Design review of the part built by this model. Coordinates are the model's own, in mm. A direction names the side the tool comes from. Give positions to 0.01 mm unless a question says otherwise; leave off trailing zeros. Write each loop counter-clockwise with the first axis right and the second up, starting at its lowest first coordinate (ties: lowest second). Pieces come first, ordered by that corner, then holes. Notation, with made-up numbers: (-7, -38.5) -> (35, -38.5) arc R21 cw to (35, -22.5) -> close; hole circle Ø5 at (-18.75, -12.75). An arc over 180 degrees is marked (long way). Put each result on its own line as item: value. Start each with the question number.
from build123d import *

# Parameters (mm, degrees)
SKETCH1_R           = 13
BOSS_EXTRUDE1_DEPTH = 17.5
SKETCH6_R           = 5
BOSS_EXTRUDE2_DEPTH = 6
SKETCH7_R           = 5.5
BOSS_EXTRUDE3_DEPTH = 0.5
SKETCH2_R           = 1.65
CUT_EXTRUDE1_DEPTH  = 24.5
CUT_EXTRUDE3_START  = -4
SKETCH5_R           = 3.55
CUT_EXTRUDE3_DEPTH  = 11
CIRPATTERN1_COUNT   = 4
SKETCH3_R           = 2.05
CUT_EXTRUDE2_DEPTH  = 24.5
SKETCH8_R           = 2.75
CUT_EXTRUDE4_DEPTH  = 10
CUT_EXTRUDE5_DEPTH  = 10


with BuildPart() as part:
    # Sketch1 → Boss-Extrude1 (new body)
    with BuildSketch(Plane(origin=(0, 0, 0), x_dir=(1, 0, 0), z_dir=(0, 1, 0))):
        Circle(SKETCH1_R)
    extrude(amount=BOSS_EXTRUDE1_DEPTH)

    # Sketch6 → Boss-Extrude2 (add)
    with BuildSketch(Plane(origin=(0, 17.5, 0), x_dir=(1, 0, 0), z_dir=(0, 1, 0))):
        with Locations((1, 0)):
            Circle(SKETCH6_R)
    extrude(amount=BOSS_EXTRUDE2_DEPTH)

    # Sketch7 → Boss-Extrude3 (add)
    with BuildSketch(Plane(origin=(0, 17.5, 0), x_dir=(1, 0, 0), z_dir=(0, 1, 0))):
        with Locations((1, 0)):
            Circle(SKETCH7_R)
    extrude(amount=BOSS_EXTRUDE3_DEPTH)

    # Sketch2 → Cut-Extrude1 (cut, through all)
    with BuildSketch(Plane(origin=(0, 0, 0), x_dir=(1, 0, 0), z_dir=(0, 1, 0))):
        with Locations((0, 9)):
            Circle(SKETCH2_R)
    cut_extrude1 = extrude(amount=CUT_EXTRUDE1_DEPTH, mode=Mode.SUBTRACT)

    # Sketch5 → Cut-Extrude3 (cut)
    with BuildSketch(Plane(origin=(0, 17.5, 0), x_dir=(1, 0, 0), z_dir=(0, 1, 0)).offset(CUT_EXTRUDE3_START)):
        with Locations((0, 9)):
            Circle(SKETCH5_R)
    cut_extrude3 = extrude(amount=CUT_EXTRUDE3_DEPTH, mode=Mode.SUBTRACT)

    # CirPattern1: Cut-Extrude1, Cut-Extrude3 ×4 about axis
    cirpattern1_axis = Axis((0, 0, 0), (0, 1, 0))
    for i in range(1, CIRPATTERN1_COUNT):
        add(cut_extrude1.rotate(cirpattern1_axis, i * 360 / CIRPATTERN1_COUNT), mode=Mode.SUBTRACT)
        add(cut_extrude3.rotate(cirpattern1_axis, i * 360 / CIRPATTERN1_COUNT), mode=Mode.SUBTRACT)

    # Sketch3 → Cut-Extrude2 (cut, through all)
    with BuildSketch(Plane(origin=(0, 0, 0), x_dir=(1, 0, 0), z_dir=(0, 1, 0))):
        Circle(SKETCH3_R)
    extrude(amount=CUT_EXTRUDE2_DEPTH, mode=Mode.SUBTRACT)

    # Sketch8 → Cut-Extrude4 (cut)
    with BuildSketch(Plane.XZ):
        Circle(SKETCH8_R)
    extrude(amount=-CUT_EXTRUDE4_DEPTH, mode=Mode.SUBTRACT)

    # Sketch10 → Cut-Extrude5 (cut)
    with BuildSketch(Plane.XZ):
        Polygon((4.618802154, 0), (2.309401077, 4), (-2.309401077, 4), (-4.618802154, 0), (-2.309401077, -4), (2.309401077, -4), align=None)
    extrude(amount=-CUT_EXTRUDE5_DEPTH, mode=Mode.SUBTRACT)


solid = part.part
Q1. Take a section at D-D on y = 13. Give the boundary of the cut face in (x, z).
Q2. Mouldability with a two-part tool opening along X and no side actions: class faces 1 (the face through (-4, 21, 0)), 2 (the face through (-3.9, 18, -1.7)), 3 (the face through (-3.448, 4.93, 2.028)) as +X half, -X half, draft (parallel to the pull), parting line (faces both ways), or undercut.
Q3. Machinability: for faces 4 (the face through (-0.77, 15.472, -5.534)), 5 (the face through (0.4, 6.7, 7.4)), which of the approach directions +Z, -Z, +X, -X, +Y, -Y give a long, thin tool a straight path to every point of the face, cutting with its end or side? Answer none if there is none.
Q4. Take a section at A-A on y = 9.5. Give the boundary of the cut face in (x, z).
Q5. Take a section at C-C on z = 6. Give the boundary of the cut face in (x, y), then the cut area to 3 significant figures.
Q6. For pin 1 (8 mm diameter, centred on x = -10.5, z = -1, fed in from +Y); pin 2 (12 mm diameter, centred on y = 5, z = -7, fed in from -X); pin 3 (3 mm diameter, centred on x = 0, z = -9, fed in from -Y); pin 4 (1.5 mm diameter, centred on x = 3, y = 11, fed in from +Z), all flat-tipped, find the tip position at first contact; note any pin that passes through.
Q7. Take a section at B-B on x = -9.5. Give the boundary of the cut face in (y, z).
Q8. To check wall thickness, follow probe 1 along Z at (x, y) = (0, 14.3); probe 2 along X at (y, z) = (12, 1.5); probe 3 along Y at (x, z) = (9.75, 3.75). State the ranges of each line that lie inside material, in increasing order. Write a range as from..to.
Result:
1. outline: circle Ø26 at (0, 0); hole circle Ø3.3 at (-9, 0); hole circle Ø4.1 at (0, 0); hole circle Ø3.3 at (0, -9); hole circle Ø3.3 at (0, 9); hole circle Ø3.3 at (9, 0)
2. face 1: parting line
2. face 2: draft
2. face 3: undercut
3. face 4: +Y
3. face 5: +Y, -Y
4. outline: circle Ø26 at (0, 0); hole circle Ø3.3 at (-9, 0); hole (-4.62, 0) -> (-2.31, -4) -> (2.31, -4) -> (4.62, 0) -> (2.31, 4) -> (-2.31, 4) -> close; hole circle Ø3.3 at (0, -9); hole circle Ø3.3 at (0, 9); hole circle Ø3.3 at (9, 0)
5. outline: (-11.53, 0) -> (11.53, 0) -> (11.53, 17.5) -> (1.9, 17.5) -> (1.9, 13.5) -> (-1.9, 13.5) -> (-1.9, 17.5) -> (-11.53, 17.5) -> close
5. area: 388 mm^2
6. pin 1: stops at y = 17.5
6. pin 2: stops at x = -12.96
6. pin 3: passes through
6. pin 4: stops at z = 12.8
7. outline: (0, -8.87) -> (17.5, -8.87) -> (17.5, -3.51) -> (13.5, -3.51) -> (13.5, -1.57) -> (0, -1.57) -> close; (0, 1.57) -> (13.5, 1.57) -> (13.5, 3.51) -> (17.5, 3.51) -> (17.5, 8.87) -> (0, 8.87) -> close
8. probe 1: z = -13..-12.55, -5.45..-2.05, 2.05..5.45, 12.55..13
8. probe 2: x = -12.91..-9.69, -8.31..-1.4, 1.4..8.31, 9.69..12.91
8. probe 3: y = 0..17.5
